```python
from build123d import *

# Parameters (mm, degrees)
F0_W     = 50.8
F0_H     = 12.7
F1_DEPTH = 101.6
F3_DEPTH = 101.6
F5_DEPTH = 101.6
F6_T     = -2.54


with BuildPart() as f1:
    # F0 (on Front) → F1 (new body)
    with BuildSketch(Plane.XZ):
        with Locations((25.4, 6.35)):
            Rectangle(F0_W, F0_H)
    extrude(amount=-F1_DEPTH)

    # F2 (on face) → F3 (cut)
    with BuildSketch(Plane.XZ):
        Polygon((0, 12.7), (0, 0), (19.05, 0), align=None)
    extrude(amount=-F3_DEPTH, mode=Mode.SUBTRACT)

    # F4 (on face) → F5 (cut)
    with BuildSketch(Plane.XZ):
        Polygon((31.75, 0), (50.8, 0), (50.8, 12.7), align=None)
    extrude(amount=-F5_DEPTH, mode=Mode.SUBTRACT)

    # F6
    f6_openings = [f1.faces().sort_by_distance(p)[0] for p in [
        (25.4, 50.8, 12.7),
    ]]
    offset(amount=F6_T, openings=f6_openings)


solid = f1.part
```
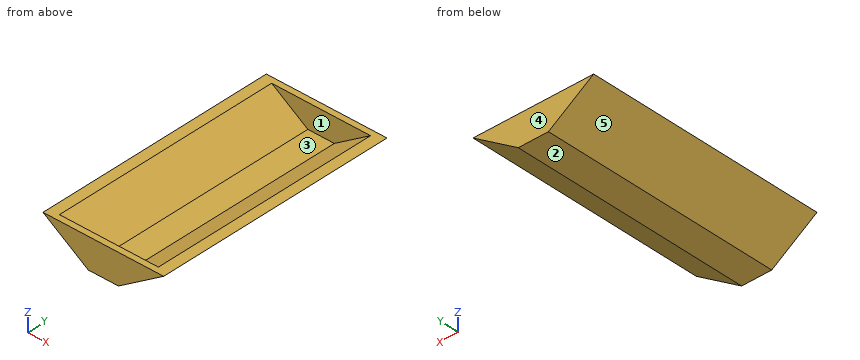
Work out the finished part from the listing and answer in its coordinate system (mm). Face numbers are marked on the shaded views. A direction names the side the tool comes from. Coordinates: 2 decimals unless noted, no trailing zeros. Loops run counter-clockwise (first coordinate to the right, second up) from the corner with the lowest first, then second, coordinate; pieces in that order, holes last.
1) Section D-D (z = 6) is taken. Give the vertices of the cut face in (x, y), plus the area to 3 significant figures.
Results:
outline: (10.05, 0) - (40.75, 0) - (40.75, 101.6) - (10.05, 101.6) - close; hole (14.63, 2.54) - (36.17, 2.54) - (36.17, 99.06) - (14.63, 99.06) - close
area: 1,040 mm2
2) For the marked faces 1 and 2, determine the directions among +Z, -Z, +X, -X, +Y, -Y from which every point of the face is accessible in a straight line to the end or side of a thin tool.
Results:
face 1: +Z
face 2: -Z, +X, -X, +Y, -Y
3) For a pull along X with two mould halves and no side action, classify the marked faces 3, 4 and 5 as +X half, -X half, draft (parallel to the pull), parting line (faces both ways), or undercut.
Results:
face 3: undercut
face 4: draft
face 5: -X half
4) Section B-B (x = 26.5) is taken. Give the vertices of the cut face in (y, z).
Results:
outline: (0, 0) - (101.6, 0) - (101.6, 12.7) - (99.06, 12.7) - (99.06, 2.54) - (2.54, 2.54) - (2.54, 12.7) - (0, 12.7) - close
5) Section A-A (y = 47.5) is taken. Give the vertices of the cut face in (x, z), plus the area to 3 significant figures.
Results:
outline: (0, 12.7) - (19.05, 0) - (31.75, 0) - (50.8, 12.7) - (46.22, 12.7) - (30.98, 2.54) - (19.82, 2.54) - (4.58, 12.7) - close
area: 135 mm2
6) Flat-ended cylindrical pins translate along their axes: pin 1 (4 mm diameter, centred on y = 63.5, z = 5, fed in from -X); pin 2 (6 mm diameter, centred on y = 16.5, z = 8, fed in from +X); pin 3 (12.5 mm diameter, centred on x = 27, y = 35.5, fed in from +Z). Find the tip coordinate at first contact, or state that the pin passes through.
Results:
pin 1: stops at x = 8.55
pin 2: stops at x = 48.25
pin 3: stops at z = 4.05
7) Section C-C (z = 11.25) is taken. Give the vertices of the cut face in (x, y) (3 decimals).
Results:
outline: (2.175, 0) - (48.625, 0) - (48.625, 101.6) - (2.175, 101.6) - close; hole (6.754, 2.54) - (44.046, 2.54) - (44.046, 99.06) - (6.754, 99.06) - close
8) Consider probe 1 along Y at (x, z) = (27.5, 12); probe 2 along Z at (x, y) = (27, 23); probe 3 along X at (y, z) = (71.5, 11.25) (3 decimals). Determine where each line is inside the solid, lowest interval first.
Results:
probe 1: y = 0 to 2.54, 99.06 to 101.6
probe 2: z = 0 to 2.54
probe 3: x = 2.175 to 6.754, 44.046 to 48.625
